Design review of the part built by this model. Coordinates are the model's own, in mm. A direction names the side the tool comes from. Give positions to 0.01 mm unless a question says otherwise; leave off trailing zeros. Loops run counter-clockwise (first coordinate to the right, second up) from the corner with the lowest first, then second, coordinate; pieces in that order, holes last. Notation, with made-up numbers: (17, 88.25) - (36, 88.25) arc R34 ccw to (36, 118.25) - close; hole circle Ø10 at (28, -19). An arc over 180 degrees is marked (long way). Write each question's results on one line, items separated by ' | '.
from build123d import *

# Parameters (mm, degrees)
SKETCH1_W           = 127
SKETCH1_H           = 63.5
BOSS_EXTRUDE1_DEPTH = 5.08
SKETCH2_W           = 127
SKETCH2_H           = 63.5
SKETCH2_W_2         = 121.92
SKETCH2_H_2         = 58.42
BOSS_EXTRUDE3_DEPTH = 38.1
CUT_EXTRUDE1_REACH  = 150.411
SKETCH3_R           = 12.7
SKETCH3_R_2         = 2.159
CUT_EXTRUDE3_REACH  = 150.411
SKETCH4_R           = 3.175
FILLET3_R           = 5.08
FILLET4_R           = 2.54


with BuildPart() as part:
    # Sketch1 → Boss-Extrude1 (new body)
    with BuildSketch(Plane(origin=(0, 0, 0), x_dir=(1, 0, 0), z_dir=(0, 1, 0))):
        with Locations((63.5, 31.75)):
            Rectangle(SKETCH1_W, SKETCH1_H)
    extrude(amount=BOSS_EXTRUDE1_DEPTH)

    # Sketch2 → Boss-Extrude3 (add)
    with BuildSketch(Plane(origin=(0, 5.08, 0), x_dir=(1, 0, 0), z_dir=(0, 1, 0))):
        with Locations((63.5, 31.75)):
            Rectangle(SKETCH2_W, SKETCH2_H)
        with Locations((63.5, 31.75)):
            Rectangle(SKETCH2_W_2, SKETCH2_H_2, mode=Mode.SUBTRACT)
    extrude(amount=BOSS_EXTRUDE3_DEPTH)

    # Sketch3 → Cut-Extrude1 (cut, up to next)
    with BuildSketch(Plane.ZY, mode=Mode.PRIVATE) as cut_extrude1_sk1:
        with Locations((-31.75, 24.13)):
            Circle(SKETCH3_R)
    cut_extrude1_tool1 = extrude(cut_extrude1_sk1.sketch, amount=-CUT_EXTRUDE1_REACH, mode=Mode.PRIVATE) & part.part
    # Sketch3 → Cut-Extrude1 (cut, up to next)
    with BuildSketch(Plane.ZY, mode=Mode.PRIVATE) as cut_extrude1_sk2:
        with Locations((-46.9265, 35.3568)):
            Circle(SKETCH3_R_2)
    cut_extrude1_tool2 = extrude(cut_extrude1_sk2.sketch, amount=-CUT_EXTRUDE1_REACH, mode=Mode.PRIVATE) & part.part
    # Sketch3 → Cut-Extrude1 (cut, up to next)
    with BuildSketch(Plane.ZY, mode=Mode.PRIVATE) as cut_extrude1_sk3:
        with Locations((-16.5735, 35.3568)):
            Circle(SKETCH3_R_2)
    cut_extrude1_tool3 = extrude(cut_extrude1_sk3.sketch, amount=-CUT_EXTRUDE1_REACH, mode=Mode.PRIVATE) & part.part
    # Sketch3 → Cut-Extrude1 (cut, up to next)
    with BuildSketch(Plane.ZY, mode=Mode.PRIVATE) as cut_extrude1_sk4:
        with Locations((-46.9265, 12.9032)):
            Circle(SKETCH3_R_2)
    cut_extrude1_tool4 = extrude(cut_extrude1_sk4.sketch, amount=-CUT_EXTRUDE1_REACH, mode=Mode.PRIVATE) & part.part
    # Sketch3 → Cut-Extrude1 (cut, up to next)
    with BuildSketch(Plane.ZY, mode=Mode.PRIVATE) as cut_extrude1_sk5:
        with Locations((-16.5735, 12.9032)):
            Circle(SKETCH3_R_2)
    cut_extrude1_tool5 = extrude(cut_extrude1_sk5.sketch, amount=-CUT_EXTRUDE1_REACH, mode=Mode.PRIVATE) & part.part
    add(cut_extrude1_tool1.solids().sort_by_distance((0, 24.13, -31.75))[0], mode=Mode.SUBTRACT)
    add(cut_extrude1_tool2.solids().sort_by_distance((0, 35.3568, -46.9265))[0], mode=Mode.SUBTRACT)
    add(cut_extrude1_tool3.solids().sort_by_distance((0, 35.3568, -16.5735))[0], mode=Mode.SUBTRACT)
    add(cut_extrude1_tool4.solids().sort_by_distance((0, 12.9032, -46.9265))[0], mode=Mode.SUBTRACT)
    add(cut_extrude1_tool5.solids().sort_by_distance((0, 12.9032, -16.5735))[0], mode=Mode.SUBTRACT)

    # Sketch4 → Cut-Extrude3 (cut, up to next)
    with BuildSketch(Plane(origin=(127, 0, 0), x_dir=(0, 0, -1), z_dir=(1, 0, 0)), mode=Mode.PRIVATE) as cut_extrude3_sk1:
        with Locations((31.75, 15.24)):
            Circle(SKETCH4_R)
    cut_extrude3_tool1 = extrude(cut_extrude3_sk1.sketch, amount=-CUT_EXTRUDE3_REACH, mode=Mode.PRIVATE) & part.part
    add(cut_extrude3_tool1.solids().sort_by_distance((127, 15.24, -31.75))[0], mode=Mode.SUBTRACT)

    # Fillet3
    fillet3_edges = [part.edges().sort_by_distance(p)[0] for p in [
        (0, 21.59, -63.5),
        (127, 21.59, -63.5),
        (127, 21.59, 0),
        (0, 21.59, 0),
    ]]
    fillet(fillet3_edges, radius=FILLET3_R)

    # Fillet4
    fillet4_edges = [part.edges().sort_by_distance(p)[0] for p in [
        (2.54, 24.13, -2.54),
        (124.46, 24.13, -2.54),
        (124.46, 24.13, -60.96),
        (2.54, 24.13, -60.96),
    ]]
    fillet(fillet4_edges, radius=FILLET4_R)


solid = part.part
(1) Tool access review of faces 1 (the flat face through (2.54, 19.6, -19.5)), 2 (the cylindrical face through (1.25, 33.25, -47.39)), 3 (the flat face through (63, 0, -32)): name each direction out of +Z, -Z, +X, -X, +Y, -Y from which nothing blocks a thin tool from reaching the whole face with its end or side.
Answers below:
face 1: +Y | face 2: -X | face 3: +Z, -Z, +X, -X, -Y
(2) Draft analysis for pull direction X (two halves, no side actions). For faces 4 (the cylindrical face through (125.472, 21.892, -1.449)), 5 (the cylindrical face through (1.449, 21.892, -1.528)), 6 (the flat face through (44, 43.18, -1)), 7 (the cylindrical face through (123.736, 24.397, -60.196)), state which applies: pulls with the +X half, pulls with the -X half, needs draft (parallel to the pull), parting line crosses it, or undercut.
Answers below:
face 4: pulls with the +X half | face 5: pulls with the -X half | face 6: needs draft | face 7: undercut
(3) Wall thickness on line 1 along Z through (x, y) = (121, 26.5); line 2 along X through (y, z) = (22.5, -25.5); line 3 along Y through (x, z) = (37, -5): over which ranges is each line inside the solid? List them lowest first. Write a range as from..to.
Answers below:
line 1: -63.5..-60.96, -2.54..0 | line 2: 124.46..127 | line 3: 0..5.08
(4) Insertion check: P1, Ø17.5, axis at x = 62.5, z = -40, coming from the +Y side; P2, Ø3.5, axis at y = 12.9, z = -16.57, coming from the -X side. Each pin has a flat end and moves straight along its axis. Give the tip position at first contact, or say it passes through.
Answers below:
P1: y = 5.08 | P2: x = 124.46
(5) Take a section at D-D on y = 24.13. Give the boundary of the cut face in (x, z), plus the area to 3 significant figures.
Answers below:
outline: (0, -58.42) arc R5.08 ccw to (5.08, -63.5) - (121.92, -63.5) arc R5.08 ccw to (127, -58.42) - (127, -5.08) arc R5.08 ccw to (121.92, 0) - (5.08, 0) arc R5.08 ccw to (0, -5.08) - (0, -19.05) - (2.54, -19.05) - (2.54, -5.08) arc R2.54 cw to (5.08, -2.54) - (121.92, -2.54) arc R2.54 cw to (124.46, -5.08) - (124.46, -58.42) arc R2.54 cw to (121.92, -60.96) - (5.08, -60.96) arc R2.54 cw to (2.54, -58.42) - (2.54, -44.45) - (0, -44.45) - close | area: 861 mm2
(6) Take a section at C-C on x = 75. Give the boundary of the cut face in (y, z).
Answers below:
outline: (0, -63.5) - (43.18, -63.5) - (43.18, -60.96) - (5.08, -60.96) - (5.08, -2.54) - (43.18, -2.54) - (43.18, 0) - (0, 0) - close
(7) Take a section at A-A on z = -31.75. Give the boundary of the cut face in (x, y) (3 decimals).
Answers below:
outline: (0, 0) - (127, 0) - (127, 12.065) - (124.46, 12.065) - (124.46, 5.08) - (2.54, 5.08) - (2.54, 11.43) - (0, 11.43) - close; (0, 36.83) - (2.54, 36.83) - (2.54, 43.18) - (0, 43.18) - close; (124.46, 18.415) - (127, 18.415) - (127, 43.18) - (124.46, 43.18) - close
(8) Take a section at B-B on y = 8. Give the boundary of the cut face in (x, z), plus the area to 3 significant figures.
Answers below:
outline: (0, -58.42) arc R5.08 ccw to (5.08, -63.5) - (121.92, -63.5) arc R5.08 ccw to (127, -58.42) - (127, -5.08) arc R5.08 ccw to (121.92, 0) - (5.08, 0) arc R5.08 ccw to (0, -5.08) - close; hole (2.54, -58.42) arc R2.54 ccw to (5.08, -60.96) - (121.92, -60.96) arc R2.54 ccw to (124.46, -58.42) - (124.46, -5.08) arc R2.54 ccw to (121.92, -2.54) - (5.08, -2.54) arc R2.54 ccw to (2.54, -5.08) - close | area: 925 mm2
